The listing builds one solid part. Answer for the finished solid, in the listing's coordinates (mm). Face numbers are marked on the shaded views. A direction names the side the tool comes from. Coordinates: 2 decimals unless noted, no trailing zeros. Loops run counter-clockwise (first coordinate to the right, second up) from the corner with the lowest first, then second, coordinate; pieces in that order, holes last. Notation, with made-up numbers: M 35,75.25 L 52,75.25 A24 ccw 52,109.25 Z; hole C -11,63.5 d4. An arc over 180 degrees is marked long. Answer in a Markdown table with one row per item. Add a question column.
from build123d import *

# Parameters (mm, degrees)
SKETCH1_W           = 40
SKETCH1_H           = 50
BOSS_EXTRUDE1_DEPTH = 5
SKETCH2_W           = 5
SKETCH2_H           = 50
BOSS_EXTRUDE2_DEPTH = 25
SKETCH3_R           = 4
CUT_EXTRUDE1_DEPTH  = 56.901699437
SKETCH4_W           = 5
SKETCH4_H           = 30
BOSS_EXTRUDE3_DEPTH = 20
SKETCH5_R           = 3
BOSS_EXTRUDE4_DEPTH = 5
SKETCH6_R           = 15
BOSS_EXTRUDE5_DEPTH = 30


with BuildPart() as part:
    # Sketch1 → Boss-Extrude1 (new body)
    with BuildSketch(Plane.XY):
        Rectangle(SKETCH1_W, SKETCH1_H)
    extrude(amount=BOSS_EXTRUDE1_DEPTH)

    # Sketch2 → Boss-Extrude2 (add)
    with BuildSketch(Plane.XY.offset(5)):
        with Locations((-17.5, 0)):
            Rectangle(SKETCH2_W, SKETCH2_H)
        with Locations((17.5, 0)):
            Rectangle(SKETCH2_W, SKETCH2_H)
    extrude(amount=BOSS_EXTRUDE2_DEPTH)

    # Sketch3 → Cut-Extrude1 (cut, through all)
    with BuildSketch(Plane.ZY.offset(20)):
        with Locations((20, 0)):
            Circle(SKETCH3_R)
    extrude(amount=-CUT_EXTRUDE1_DEPTH, mode=Mode.SUBTRACT)

    # Sketch4 → Boss-Extrude3 (add)
    with BuildSketch(Plane.ZY.offset(20)):
        with Locations((2.5, 0)):
            Rectangle(SKETCH4_W, SKETCH4_H)
    extrude(amount=BOSS_EXTRUDE3_DEPTH)

    # Sketch5 → Boss-Extrude4 (add)
    with BuildSketch(Plane.XY.offset(5)):
        with BuildLine():
            Line((-40, 15), (-77.785894763, 62.179423312))
            ThreePointArc((-77.785894763, 62.179423312), (-88.196441443, 63.448140197), (-89.697194155, 53.068503112))
            Line((-89.697194155, 53.068503112), (-40, -15))
            Line((-40, -15), (-40, 15))
        make_face()
        with Locations((-83.639846307, 57.491006594)):
            Circle(SKETCH5_R, mode=Mode.SUBTRACT)
    extrude(amount=-BOSS_EXTRUDE4_DEPTH)

    # Sketch6 → Boss-Extrude5 (add)
    with BuildSketch(Plane(origin=(0, 0, 0), x_dir=(-1, 0, 0), z_dir=(0, 0, -1))):
        Circle(SKETCH6_R)
    extrude(amount=BOSS_EXTRUDE5_DEPTH)


with BuildPart() as body_2:
    # Mirror1: mirrored copy
    add(part.part.mirror(Plane(origin=(0, 0, -30), x_dir=(1, 0, 0), z_dir=(0, 0, -1))))


solid = body_2.part
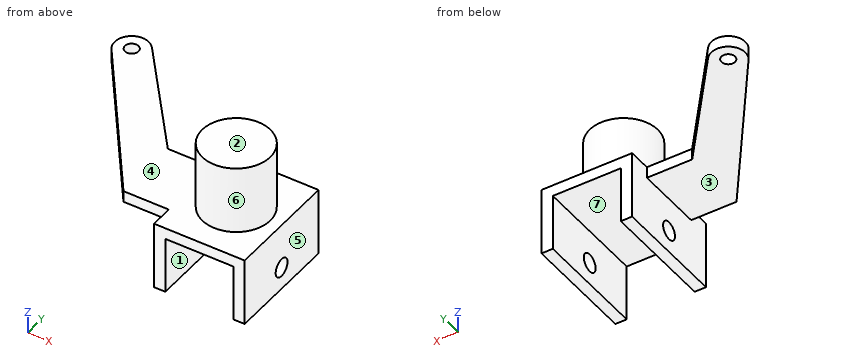
(1) A cutting plane is placed at D-D (z = -80). Give the vertices of the cut face in (x, y).
(2) Each of these flat-tipped pins is pushed along its axis until it touches: pin 1 (2 mm diameter, centred on x = -23, y = -14.5, fed in from -Z); pin 2 (5.5 mm diameter, centred on x = -33, z = -63.5, fed in from +Y); pin 3 (20 mm diameter, centred on y = -2, z = -79.5, fed in from -X). Where does it stop, or does it pass through?
(3) The mould has two halves that part along X. Classify the marked faces 4, 5, 6 and 7: released by +X, released by -X, zero draft, split by the parting line, or undercut.
(4) A cutting plane is placed at B-B (y = -1.5). Give the vertices of the cut face in (x, z).
(5) For the marked faces 1, 2 and 3, determine the directions among +Z, -Z, +X, -X, +Y, -Y from which every point of the face is accessible in a straight line to the end or side of a thin tool.
(6) Straight lines are drawn through the part: line 1 (X direction, y = -3.5, z = -76); line 2 (Y direction, x = 16.9, z = -80); line 3 (Z direction, x = 0, y = 17.5). For each, find the intervals that lie inside material, in ascending order.
(7) A cutting plane is placed at A-A (z = -72). Give the vertices of the cut face in (x, y), plus the area to 3 significant figures.
(8) A cutting plane is placed at C-C (x = 0). Give the vertices of the cut face in (y, z).
Solved:
| question | item | result |
|---|---|---|
| 1 | outline | M -20,-25 L -15,-25 L -15,-4 L -20,-4 Z; M -20,4 L -15,4 L -15,25 L -20,25 Z; M 15,-25 L 20,-25 L 20,-4 L 15,-4 Z; M 15,4 L 20,4 L 20,25 L 15,25 Z |
| 2 | pin 1 | stops at z = -65 |
| 2 | pin 2 | stops at y = 15 |
| 2 | pin 3 | stops at x = -20 |
| 3 | face 4 | zero draft |
| 3 | face 5 | released by +X |
| 3 | face 6 | split by the parting line |
| 3 | face 7 | undercut |
| 4 | outline | M -49.86,-65 L -20,-65 L -20,-76.29 L -15,-76.29 L -15,-65 L 15,-65 L 15,-76.29 L 20,-76.29 L 20,-60 L 14.92,-60 L 14.92,-30 L -14.92,-30 L -14.92,-60 L -49.86,-60 Z; M -20,-90 L -15,-90 L -15,-83.71 L -20,-83.71 Z; M 15,-90 L 20,-90 L 20,-83.71 L 15,-83.71 Z |
| 5 | face 1 | -Z, +Y, -Y |
| 5 | face 2 | +Z, +X, -X, +Y, -Y |
| 5 | face 3 | -Z, -X, +Y, -Y |
| 6 | line 1 | x = -20 to -15, 15 to 20 |
| 6 | line 2 | y = -25 to -4, 4 to 25 |
| 6 | line 3 | z = -65 to -60 |
| 7 | outline | M -20,-25 L -15,-25 L -15,25 L -20,25 Z; M 15,-25 L 20,-25 L 20,25 L 15,25 Z |
| 7 | area | 500 mm² |
| 8 | outline | M -25,-65 L 25,-65 L 25,-60 L 15,-60 L 15,-30 L -15,-30 L -15,-60 L -25,-60 Z |
